Geometry check sheet. Reference: drawing and pictorial views, mm from the part's lowest x, y, z. Coordinates: 2 decimals unless noted, no trailing zeros. Loops run counter-clockwise (first coordinate to the right, second up) from the corner with the lowest first, then second, coordinate; pieces in that order, holes last. Notation, with made-up numbers: M -14.75,87 L 10.25,87 A30 cw 10.25,122 Z; hole C 10,48.25 d6. An arc over 180 degrees is marked long. Write each question's results on one line, items separated by ' | '. Start each with the question number.
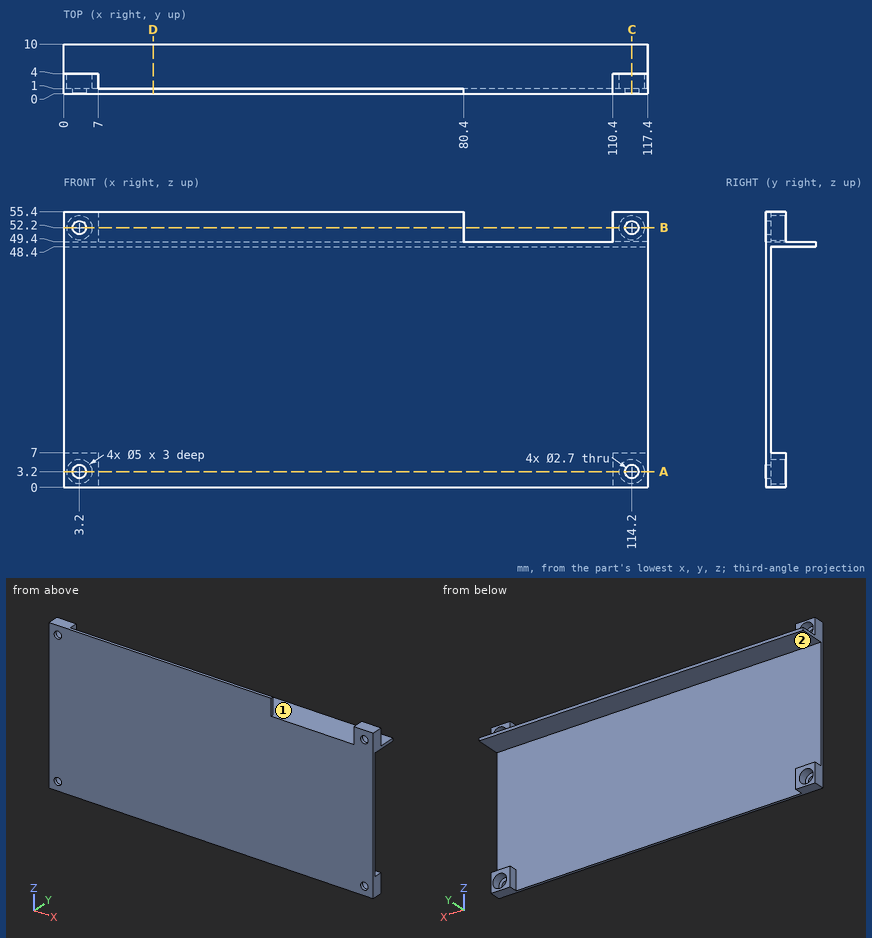
1) Release check for a two-part mould opening along X. For the marked faces 1 and 2 record: +X half, -X half, draft (parallel to the pull), parting line (faces both ways), or undercut.
2) Thickness scan on probe 1 along X at (y, z) = (2.1, 3.2); probe 2 along X at (y, z) = (0.6, 52.2); probe 3 along Z at (x, y) = (114.2, 2.4). Record the ranges inside material, lowest first.
3) Section check C-C (x = 114.2). Enter the section's corners in (y, z).
4) Section check A-A (z = 3.2). Enter the section's corners in (x, y), then the cut area to 3 significant figures.
5) Gauge pin test, flat ends, axial feed: P1, Ø4, axis at x = 2, z = 2.5, coming from the +Y side; P2, Ø5, axis at x = 57.5, z = 51.5, coming from the +Y side; P3, Ø1, axis at x = 81.5, z = 39, coming from the +Y side; P4, Ø6, axis at x = 53.5, y = 4.5, coming from the -Z side. Record the tip position at first contact, or that the pin passes through.
6) Section check D-D (x = 18). Enter the section's corners in (y, z), then the cut area to 3 significant figures.
7) Section check B-B (z = 52.2). Enter the section's corners in (x, y).
Return value:
1) face 1: undercut | face 2: draft
2) probe 1: x = 0 to 0.7, 5.7 to 7, 110.4 to 111.7, 116.7 to 117.4 | probe 2: x = 0 to 1.85, 4.55 to 80.4, 110.4 to 112.85, 115.55 to 117.4 | probe 3: z = 0 to 0.7, 5.7 to 7, 48.4 to 49.7, 54.7 to 55.4
3) outline: M 0,0 L 4,0 L 4,0.7 L 1,0.7 L 1,1.85 L 0,1.85 Z; M 0,4.55 L 1,4.55 L 1,5.7 L 4,5.7 L 4,7 L 1,7 L 1,48.4 L 10,48.4 L 10,49.4 L 4,49.4 L 4,49.7 L 1,49.7 L 1,50.85 L 0,50.85 Z; M 0,53.55 L 1,53.55 L 1,54.7 L 4,54.7 L 4,55.4 L 0,55.4 Z
4) outline: M 0,0 L 1.85,0 L 1.85,1 L 0.7,1 L 0.7,4 L 0,4 Z; M 4.55,0 L 112.85,0 L 112.85,1 L 111.7,1 L 111.7,4 L 110.4,4 L 110.4,1 L 7,1 L 7,4 L 5.7,4 L 5.7,1 L 4.55,1 Z; M 115.55,0 L 117.4,0 L 117.4,4 L 116.7,4 L 116.7,1 L 115.55,1 Z | area: 124 mm2
5) P1: stops at y = 4 | P2: stops at y = 10 | P3: stops at y = 1 | P4: stops at z = 48.4
6) outline: M 0,0 L 1,0 L 1,48.4 L 10,48.4 L 10,49.4 L 1,49.4 L 1,55.4 L 0,55.4 Z | area: 64.4 mm2
7) outline: M 0,0 L 1.85,0 L 1.85,1 L 0.7,1 L 0.7,4 L 0,4 Z; M 4.55,0 L 80.4,0 L 80.4,1 L 7,1 L 7,4 L 5.7,4 L 5.7,1 L 4.55,1 Z; M 110.4,0 L 112.85,0 L 112.85,1 L 111.7,1 L 111.7,4 L 110.4,4 Z; M 115.55,0 L 117.4,0 L 117.4,4 L 116.7,4 L 116.7,1 L 115.55,1 Z
